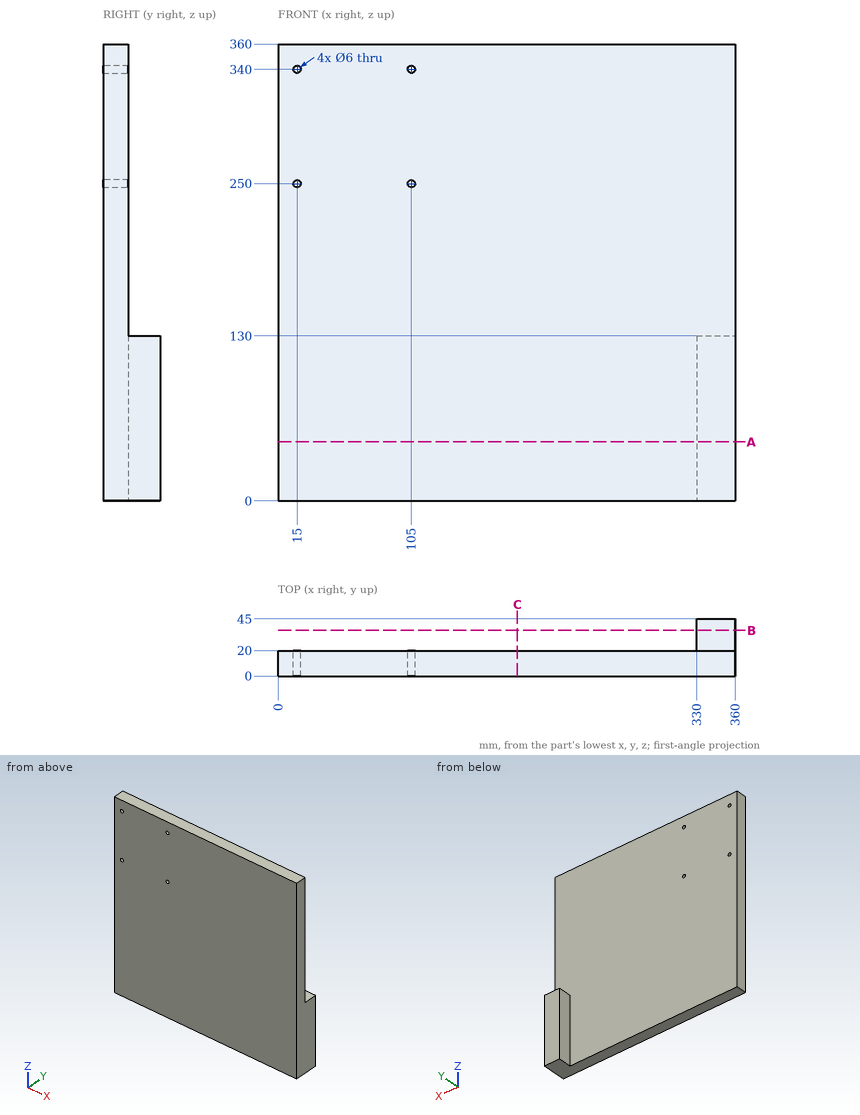
Geometry check sheet. Reference: drawing and pictorial views, mm from the part's lowest x, y, z. Give positions to 0.01 mm unless a question says otherwise; leave off trailing zeros. Write each loop counter-clockwise with the first axis right and the second up, starting at its lowest first coordinate (ties: lowest second). Pieces come first, ordered by that corner, then holes.
Item 1: Scan lines: L1, parallel to X at y = 4, z = 250; L2, parallel to Y at x = 82.5, z = 166.5; L3, parallel to X at y = 34, z = 113. Record each from-to range of solid material in increasing order.
Item 2: Cross-section at B-B (y = 36). Enter the section's corners in (x, z).
Item 3: Gauge pin test, flat ends, axial feed: pin 1 (5 mm diameter, centred on x = 261.5, z = 145.5, fed in from +Y); pin 2 (7.5 mm diameter, centred on y = 33.5, z = 55.5, fed in from -X); pin 3 (9.5 mm diameter, centred on x = 15, z = 340, fed in from -Y). Record the tip position at first contact, or that the pin passes through.
Item 4: Cross-section at A-A (z = 46.5). Enter the section's corners in (x, y).
Item 5: Cross-section at C-C (x = 188.5). Enter the section's corners in (y, z), and give its area (3 significant figures).
Report:
1. L1: x = 0 to 12, 18 to 102, 108 to 360
1. L2: y = 0 to 20
1. L3: x = 330 to 360
2. outline: (330, 0) - (360, 0) - (360, 130) - (330, 130) - close
3. pin 1: stops at y = 20
3. pin 2: stops at x = 330
3. pin 3: stops at y = 0
4. outline: (0, 0) - (360, 0) - (360, 45) - (330, 45) - (330, 20) - (0, 20) - close
5. outline: (0, 0) - (20, 0) - (20, 360) - (0, 360) - close
5. area: 7,200 mm2
